Answer from the drawing. Dimensions are ordinates in mm from the lowest x, y and z of the part. Coordinates: 2 decimals unless noted, no trailing zeros. Loops run counter-clockwise (first coordinate to the right, second up) from the corner with the lowest first, then second, coordinate; pieces in that order, holes last. Notation, with made-up numbers: (33, -32) - (45, -32) arc R24 ccw to (45, -18) - close; hole circle Ø10 at (-12.75, 4.5). An arc over 180 degrees is marked (long way). Use one line per item in the form item = value. Start each with the question number.
1) A cutting plane is placed at D-D (x = 9). Give the vertices of the cut face in (y, z), and give its area (3 significant figures).
2) The mould has two halves that part along Z. Classify the marked faces 1, 2, 3 and 4: released by +Z, released by -Z, zero draft, split by the parting line, or undercut.
3) A cutting plane is placed at C-C (z = 3). Give the vertices of the cut face in (x, y).
4) Consider line 1 (Y direction, x = 5.25, z = 7.5); line 2 (X direction, y = 15, z = 9); line 3 (Z direction, x = 15, y = 45). Determine where each line is inside the solid, lowest interval first.
5) A cutting plane is placed at A-A (x = 13.25). Give the vertices of the cut face in (y, z), and give its area (3 significant figures).
6) Each of these flat-tipped pins is pushed along its axis until it touches: P1, Ø8, axis at y = 21, z = 12, coming from the +X side; P2, Ø3.5, axis at y = 44.63, z = 7.5, coming from the +X side (1 decimal). Where does it stop, or does it pass through?
7) A cutting plane is placed at B-B (z = 7.5). Give the vertices of the cut face in (x, y).
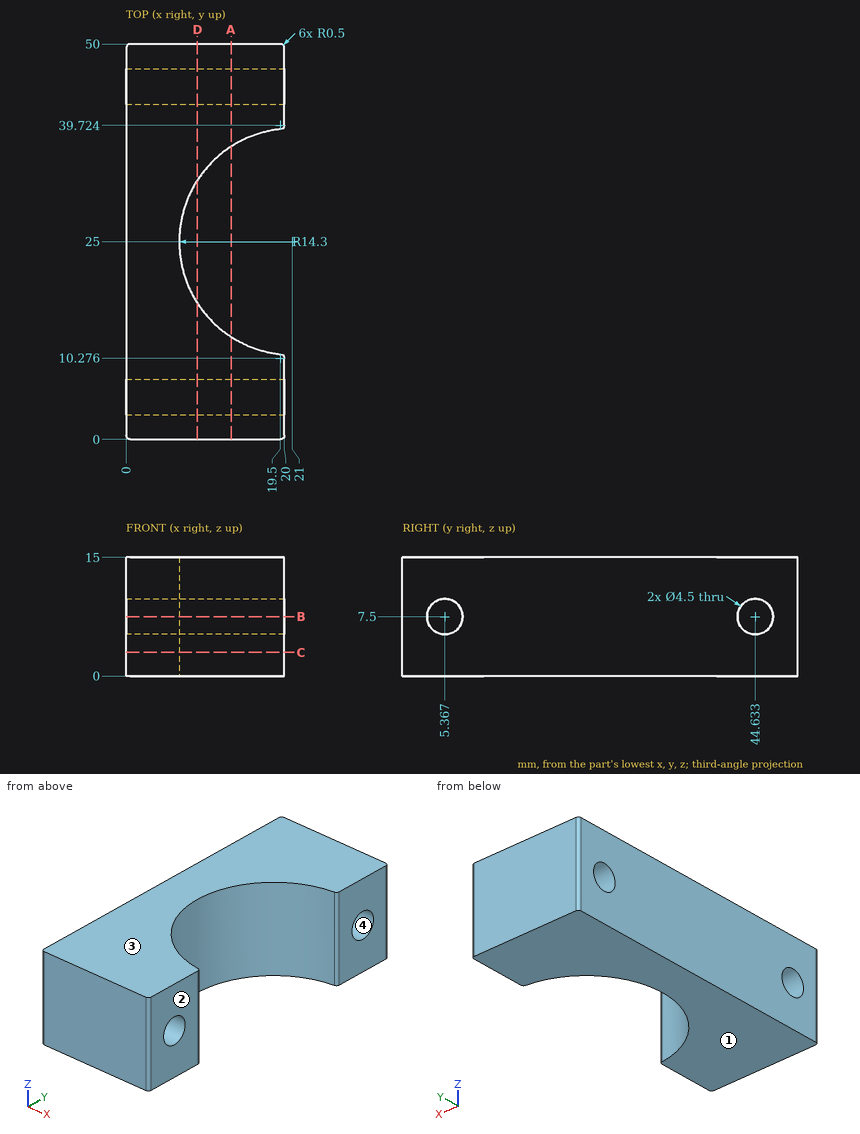
Found:
q1.outline = (0, 0) - (17.22, 0) - (17.22, 15) - (0, 15) - close; (32.78, 0) - (50, 0) - (50, 15) - (32.78, 15) - close; hole circle Ø4.5 at (5.37, 7.5); hole circle Ø4.5 at (44.63, 7.5)
q1.area = 485 mm^2
q2.face_1 = released by -Z
q2.face_2 = zero draft
q2.face_3 = released by +Z
q2.face_4 = undercut
q3.outline = (0, 0.5) arc R0.5 ccw to (0.5, 0) - (19.5, 0) arc R0.5 ccw to (20, 0.5) - (20, 10.28) arc R0.5 ccw to (19.55, 10.77) arc R14.3 cw to (19.55, 39.23) arc R0.5 ccw to (20, 39.72) - (20, 49.5) arc R0.5 ccw to (19.5, 50) - (0.5, 50) arc R0.5 ccw to (0, 49.5) - close
q4.line_1 = 0 to 3.12, 7.62 to 42.38, 46.88 to 50
q4.line_2 = 0 to 10.78
q4.line_3 = 0 to 5.28, 9.72 to 15
q5.outline = (0, 0) - (12.98, 0) - (12.98, 15) - (0, 15) - close; (37.02, 0) - (50, 0) - (50, 15) - (37.02, 15) - close; hole circle Ø4.5 at (5.37, 7.5); hole circle Ø4.5 at (44.63, 7.5)
q5.area = 358 mm^2
q6.P1 = 9.15
q6.P2 = through
q7.outline = (0, 0.5) arc R0.5 ccw to (0.5, 0) - (19.5, 0) arc R0.5 ccw to (20, 0.5) - (20, 3.12) - (0, 3.12) - close; (0, 7.62) - (20, 7.62) - (20, 10.28) arc R0.5 ccw to (19.55, 10.77) arc R14.3 cw to (19.55, 39.23) arc R0.5 ccw to (20, 39.72) - (20, 42.38) - (0, 42.38) - close; (0, 46.88) - (20, 46.88) - (20, 49.5) arc R0.5 ccw to (19.5, 50) - (0.5, 50) arc R0.5 ccw to (0, 49.5) - close
